from build123d import *

# Parameters (mm, degrees)
SKETCH1_W           = 50.8
SKETCH1_H           = 25.4
SKETCH1_W_2         = 44.45
SKETCH1_H_2         = 19.05
BOSS_EXTRUDE1_DEPTH = 728.3704
CUT_EXTRUDE1_DEPTH  = 730.255620202
CUT_EXTRUDE2_DEPTH  = 728.6244


with BuildPart() as part:
    # Sketch1 → Boss-Extrude1 (new body)
    with BuildSketch(Plane(origin=(0, 0, 0), x_dir=(1, 0, 0), z_dir=(0, 1, 0))):
        Rectangle(SKETCH1_W, SKETCH1_H)
        Rectangle(SKETCH1_W_2, SKETCH1_H_2, mode=Mode.SUBTRACT)
    extrude(amount=BOSS_EXTRUDE1_DEPTH)

    # Sketch2 → Cut-Extrude1 (cut, through all)
    with BuildSketch(Plane.XY.offset(12.7)):
        Polygon((25.4, 728.3704), (-25.4, 728.3704), (25.4, 677.5704), align=None)
        Polygon((11.4046, 0), (-25.4, 36.8046), (-25.4, 0), align=None)
        Polygon((25.4, 0), (25.4, 13.9954), (11.4046, 0), align=None)
    extrude(amount=-CUT_EXTRUDE1_DEPTH, mode=Mode.SUBTRACT)

    # Sketch3 → Cut-Extrude2 (cut)
    with BuildSketch(Plane(origin=(-376.8852, 376.8852, 0), x_dir=(0, 0, 1), z_dir=(-0.7071067811865563, 0.7071067811865388, 0))):
        Polygon((12.7, 497.075136813), (-12.7, 488.822176529), (-12.7, 497.075136813), align=None)
    extrude(amount=-CUT_EXTRUDE2_DEPTH, mode=Mode.SUBTRACT)


solid = part.part
CAD build for the part. Positions are in the model's coordinates, mm. A direction names the side the tool comes from. Give positions to 0.01 mm unless a question says otherwise; leave off trailing zeros. Order: outer loops, then holes, each group sorted by start corner. A loop starts at its lowest first (then second) coordinate and runs counter-clockwise, first axis right, second up. Notation, with made-up numbers: (-28.5, 2.5) -> (12.5, 2.5) arc R25 ccw to (12.5, 24.5) -> close; hole circle Ø1 at (24.25, 30). An arc over 180 degrees is marked (long way). Return JSON: item names as keys, results as strings.
Q1. Mould opens along X. For faces 3 (the face through (-22.225, 374, 0)), 4 (the face through (-25.4, 378, 0)), 5 (the face through (25.4, 341, 0)) say: pulls with the +X half, pulls with the -X half, needs draft (parallel to the pull), parting line crosses it, or undercut.
Working result:
{"face 3": "undercut", "face 4": "pulls with the -X half", "face 5": "pulls with the +X half"}
Q2. Drill centre lines: line 1 (Z direction, x = 0.5, y = 399) (3 decimals); line 2 (X direction, y = 180, z = 2.5) (3 decimals); line 3 (Y direction, x = -20, z = -10.25). Where is each one in solid material? Low to high.
Working result:
{"line 1": "-12.7 to -9.525, 9.525 to 12.7", "line 2": "-25.4 to -22.225, 22.225 to 25.4", "line 3": "31.4 to 712.42"}
Q3. Saw through at C-C (x = -12.5). Write the cut outline in (y, z) (3 decimals), then the cut area to 3 significant figures.
Working result:
{"outline": "(23.905, -12.7) -> (703.799, -12.7) -> (705.258, -9.525) -> (23.905, -9.525) -> close; (23.905, 9.525) -> (714.011, 9.525) -> (715.47, 12.7) -> (23.905, 12.7) -> close", "area": "4,350 mm²"}
Q4. Flat gauge pin, fed straight in: pin 1 (1.5 mm diameter, centred on x = 11, z = -7.5, fed in from -Y). Where does the tip first touch, or does it go through?
Working result:
{"pin 1": "through"}
Q5. Saw through at A-A (z = 1.5). Write the cut outline in (x, y) (3 decimals), then the cut area to 3 significant figures.
Working result:
{"outline": "(-25.4, 36.805) -> (-22.225, 33.63) -> (-22.225, 720.049) -> (-25.4, 723.224) -> close; (22.225, 10.82) -> (25.4, 13.995) -> (25.4, 672.424) -> (22.225, 675.599) -> close", "area": "4,280 mm²"}
Q6. Which spindle directions (+Z, -Z, +X, -X, +Y, -Y) get a long thin tool onto all of the face, cutting with end or side? Do faces 1 (the face through (-11.001, 22.406, -10.289)), 2 (the face through (22.225, 340, 0)). Say none if no direction does.
Working result:
{"face 1": "+Z, -Z, -X, -Y", "face 2": "+Y, -Y"}
Q7. Saw through at B-B (y = 149.5). Write the cut outline in (x, z) (3 decimals), then the cut area to 3 significant figures.
Working result:
{"outline": "(-25.4, -12.7) -> (25.4, -12.7) -> (25.4, 12.7) -> (-25.4, 12.7) -> close; hole (-22.225, -9.525) -> (22.225, -9.525) -> (22.225, 9.525) -> (-22.225, 9.525) -> close", "area": "444 mm²"}
